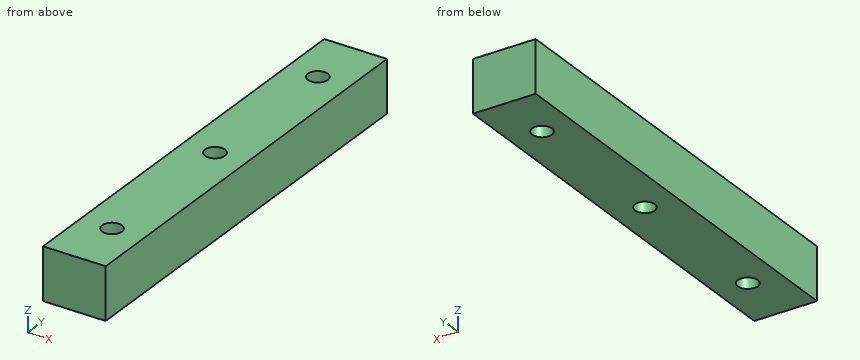
```python
from build123d import *

# Parameters (mm, degrees)
SKETCH1_W           = 29.999999944
SKETCH1_H           = 25.000000038
BOSS_EXTRUDE1_DEPTH = 204.999999956
CUT_EXTRUDE1_REACH  = 210.686
SKETCH3_R           = 4.7625


with BuildPart() as part:
    # Sketch1 → Boss-Extrude1 (new body)
    with BuildSketch(Plane(origin=(0, 0, 0), x_dir=(-1, 0, 0), z_dir=(0, 1, 0))):
        with Locations((14.999999972, 12.500000019)):
            Rectangle(SKETCH1_W, SKETCH1_H)
    extrude(amount=BOSS_EXTRUDE1_DEPTH)

    # Sketch3 → Cut-Extrude1 (cut, up to next)
    with BuildSketch(Plane(origin=(0, 0, 0), x_dir=(1, 0, 0), z_dir=(0, 0, -1)), mode=Mode.PRIVATE) as cut_extrude1_sk1:
        with Locations(Location((-14.999999972, -102.499999978, 0), (0, 0, 180))):
            Circle(SKETCH3_R)
    cut_extrude1_tool1 = extrude(cut_extrude1_sk1.sketch, amount=-CUT_EXTRUDE1_REACH, mode=Mode.PRIVATE) & part.part
    # Sketch3 → Cut-Extrude1 (cut, up to next)
    with BuildSketch(Plane(origin=(0, 0, 0), x_dir=(1, 0, 0), z_dir=(0, 0, -1)), mode=Mode.PRIVATE) as cut_extrude1_sk2:
        with Locations(Location((-14.999999972, -27.499999991, 0), (0, 0, 180))):
            Circle(SKETCH3_R)
    cut_extrude1_tool2 = extrude(cut_extrude1_sk2.sketch, amount=-CUT_EXTRUDE1_REACH, mode=Mode.PRIVATE) & part.part
    # Sketch3 → Cut-Extrude1 (cut, up to next)
    with BuildSketch(Plane(origin=(0, 0, 0), x_dir=(1, 0, 0), z_dir=(0, 0, -1)), mode=Mode.PRIVATE) as cut_extrude1_sk3:
        with Locations(Location((-14.999999972, -177.499999965, 0), (0, 0, 180))):
            Circle(SKETCH3_R)
    cut_extrude1_tool3 = extrude(cut_extrude1_sk3.sketch, amount=-CUT_EXTRUDE1_REACH, mode=Mode.PRIVATE) & part.part
    add(cut_extrude1_tool1.solids().sort_by_distance((-15, 102.5, 0))[0], mode=Mode.SUBTRACT)
    add(cut_extrude1_tool2.solids().sort_by_distance((-15, 27.5, 0))[0], mode=Mode.SUBTRACT)
    add(cut_extrude1_tool3.solids().sort_by_distance((-15, 177.5, 0))[0], mode=Mode.SUBTRACT)


solid = part.part
```
Geometry: final body of the model. Coordinates: model frame, mm. Coordinates: 2 decimals unless noted, no trailing zeros. Order: outer loops, then holes, each group sorted by start corner. A loop starts at its lowest first (then second) coordinate and runs counter-clockwise, first axis right, second up. Notation, with made-up numbers: (24.25, -36.75) - (82.25, -36.75) arc R10 ccw to (82.25, -30.75) - close; hole circle Ø7 at (4.5, 66.25). An arc over 180 degrees is marked (long way). Return JSON: item names as keys, results as strings. Group by question number.
1. Cut plane D-D (y = 175.5). Output: boundary loops of the cut face in (x, z), plus the area to 3 significant figures.
2. Cut plane C-C (z = 20.5). Output: boundary loops of the cut face in (x, y) (1 decimal).
3. Material intervals for line 1 along Y through (x, z) = (-15, 17); line 2 along X through (y, z) = (177.5, 9.5); line 3 along Y through (x, z) = (-11.5, 12), sorted ascending. Write a range as [from, to].
4. Cut plane A-A (x = -15). Output: boundary loops of the cut face in (y, z), plus the area to 3 significant figures.
5. Cut plane B-B (y = 102.5). Output: boundary loops of the cut face in (x, z), plus the area to 3 significant figures.
Resolved:
{
 "1": {"outline": "(-30, 0) - (-19.32, 0) - (-19.32, 25) - (-30, 25) - close; (-10.68, 0) - (0, 0) - (0, 25) - (-10.68, 25) - close", "area": "534 mm²"},
 "2": {"outline": "(-30, 0) - (0, 0) - (0, 205) - (-30, 205) - close; hole circle Ø9.5 at (-15, 27.5); hole circle Ø9.5 at (-15, 102.5); hole circle Ø9.5 at (-15, 177.5)"},
 "3": {"line 1": "y = [0, 22.74], [32.26, 97.74], [107.26, 172.74], [182.26, 205]", "line 2": "x = [-30, -19.76], [-10.24, 0]", "line 3": "y = [0, 24.27], [30.73, 99.27], [105.73, 174.27], [180.73, 205]"},
 "4": {"outline": "(0, 0) - (22.74, 0) - (22.74, 25) - (0, 25) - close; (32.26, 0) - (97.74, 0) - (97.74, 25) - (32.26, 25) - close; (107.26, 0) - (172.74, 0) - (172.74, 25) - (107.26, 25) - close; (182.26, 0) - (205, 0) - (205, 25) - (182.26, 25) - close", "area": "4,410 mm²"},
 "5": {"outline": "(-30, 0) - (-19.76, 0) - (-19.76, 25) - (-30, 25) - close; (-10.24, 0) - (0, 0) - (0, 25) - (-10.24, 25) - close", "area": "512 mm²"}
}
